```python
from build123d import *

# Parameters (mm, degrees)
SKETCH_W        = 12
SKETCH_H        = 77
PAD_DEPTH       = 5
PAD001_DEPTH    = 5.1
PAD002_DEPTH    = 3
SKETCH003_W     = 4
SKETCH003_H     = 105
SKETCH003_W_2   = 10
SKETCH003_H_2   = 5
PAD003_DEPTH    = 12
SKETCH004_W     = 6
SKETCH004_H     = 10
POCKET_DEPTH    = 3
POCKET001_DEPTH = 12.001
FILLET_R        = 2
PAD004_DEPTH    = 12
FILLET001_R     = 2
CHAMFER_SIZE    = 1


with BuildPart() as part:
    # Sketch → Pad (new body)
    with BuildSketch(Plane.XZ):
        with Locations((0, 38.5)):
            Rectangle(SKETCH_W, SKETCH_H)
    extrude(amount=PAD_DEPTH)

    # Sketch001 (on Face6 of Pad) → Pad001 (join)
    with BuildSketch(Plane.XZ.offset(5)):
        with BuildLine():
            Line((-2.2, 25.05), (-2.2, 22.45))
            ThreePointArc((-2.2, 22.45), (0, 20.25), (2.2, 22.45))
            Line((2.2, 25.05), (2.2, 22.45))
            ThreePointArc((2.2, 25.05), (0, 27.25), (-2.2, 25.05))
        make_face()
        with BuildLine():
            Line((-2.2, 65.05), (-2.2, 62.45))
            ThreePointArc((-2.2, 62.45), (0, 60.25), (2.2, 62.45))
            Line((2.2, 65.05), (2.2, 62.45))
            ThreePointArc((2.2, 65.05), (0, 67.25), (-2.2, 65.05))
        make_face()
    extrude(amount=PAD001_DEPTH)

    # Sketch002 (on Face16 of Pad001) → Pad002 (join)
    with BuildSketch(Plane.XZ.offset(10.1)):
        with BuildLine():
            Line((-2.2, 25.05), (-2.2, 16.45))
            ThreePointArc((-2.2, 16.45), (0, 14.25), (2.2, 16.45))
            Line((2.2, 25.05), (2.2, 16.45))
            ThreePointArc((2.2, 25.05), (0, 27.25), (-2.2, 25.05))
        make_face()
        with BuildLine():
            Line((-2.2, 65.05), (-2.2, 56.45))
            ThreePointArc((-2.2, 56.45), (0, 54.25), (2.2, 56.45))
            Line((2.2, 65.05), (2.2, 56.45))
            ThreePointArc((2.2, 65.05), (0, 67.25), (-2.2, 65.05))
        make_face()
    extrude(amount=PAD002_DEPTH)

    # Sketch003 (on Face6 of Pad002) → Pad003 (join)
    with BuildSketch(Plane(origin=(6, 0, 0), x_dir=(0, 0, 1), z_dir=(1, 0, 0))):
        with Locations((2, -52.5)):
            Rectangle(SKETCH003_W, SKETCH003_H)
        with Locations((9, -12.5)):
            Rectangle(SKETCH003_W_2, SKETCH003_H_2)
        with Locations((9, -27.5)):
            Rectangle(SKETCH003_W_2, SKETCH003_H_2)
        with Locations((9, -42.5)):
            Rectangle(SKETCH003_W_2, SKETCH003_H_2)
        with Locations((9, -57.5)):
            Rectangle(SKETCH003_W_2, SKETCH003_H_2)
        with Locations((9, -72.5)):
            Rectangle(SKETCH003_W_2, SKETCH003_H_2)
        with Locations((9, -87.5)):
            Rectangle(SKETCH003_W_2, SKETCH003_H_2)
        with Locations((9, -102.5)):
            Rectangle(SKETCH003_W_2, SKETCH003_H_2)
    extrude(amount=-PAD003_DEPTH)

    # Sketch004 (on Face30 of Pad003) → Pocket (cut)
    with BuildSketch(Plane(origin=(0, 0, 4), x_dir=(-1, 0, 0), z_dir=(0, 0, 1))):
        with Locations((0, -5)):
            Rectangle(SKETCH004_W, SKETCH004_H)
        with Locations((0, -20)):
            Rectangle(SKETCH004_W, SKETCH004_H)
        with Locations((0, -35)):
            Rectangle(SKETCH004_W, SKETCH004_H)
        with Locations((0, -50)):
            Rectangle(SKETCH004_W, SKETCH004_H)
        with Locations((0, -65)):
            Rectangle(SKETCH004_W, SKETCH004_H)
        with Locations((0, -80)):
            Rectangle(SKETCH004_W, SKETCH004_H)
        with Locations((0, -95)):
            Rectangle(SKETCH004_W, SKETCH004_H)
    extrude(amount=-POCKET_DEPTH, mode=Mode.SUBTRACT)

    # Sketch005 (on Face5 of Pocket) → Pocket001 (cut, through all)
    with BuildSketch(Plane(origin=(6, 0, 0), x_dir=(0, 0, 1), z_dir=(1, 0, 0))):
        with BuildLine():
            ThreePointArc((74.499999, 0), (77, 2.5), (74.5, 5))
            Line((74.5, 5), (77.1, 5))
            Line((77.1, 5), (77.099999, 0))
            Line((74.499999, 0), (77.099999, 0))
        make_face()
    extrude(amount=-POCKET001_DEPTH, mode=Mode.SUBTRACT)

    # Fillet
    fillet_edges = [part.edges().sort_by_distance(p)[0] for p in [
        (0, 105, 14),
        (0, 100, 14),
        (0, 90, 14),
        (0, 85, 14),
        (0, 75, 14),
        (0, 70, 14),
        (0, 60, 14),
        (0, 55, 14),
        (0, 45, 14),
        (0, 40, 14),
        (0, 30, 14),
        (0, 25, 14),
        (0, 15, 14),
        (0, 10, 14),
    ]]
    fillet(fillet_edges, radius=FILLET_R)

    # Sketch006 (on Face5 of Fillet) → Pad004 (join)
    with BuildSketch(Plane(origin=(6, 0, 0), x_dir=(0, 0, 1), z_dir=(1, 0, 0))):
        Polygon((-12, 5), (0, 5), (0, -105), align=None)
    extrude(amount=-PAD004_DEPTH)

    # Fillet001
    fillet001_edges = [part.edges().sort_by_distance(p)[0] for p in [
        (0, 105, 0),
        (0, -5, -12),
    ]]
    fillet(fillet001_edges, radius=FILLET001_R)

    # Chamfer
    chamfer_edges = [part.edges().sort_by_distance(p)[0] for p in [
        (6, -5, 32.365024),
        (6, -4.33533, -11.258877),
        (6, -4.267767, 76.267767),
        (6, 50.216895, -5.976339),
        (6, -0.732233, 76.267767),
        (6, 104.488924, 0.458354),
        (6, 0, 39.25),
        (6, 105, 6.896842),
        (6, 5, 4),
        (6, 104.414214, 13.414214),
        (6, 10, 8),
        (6, 102.5, 14),
        (6, 10.585786, 13.414214),
        (6, 100.585786, 13.414214),
        (6, 12.5, 14),
        (6, 100, 8),
        (6, 14.414214, 13.414214),
        (6, 95, 4),
        (6, 15, 8),
        (6, 90, 8),
        (6, 20, 4),
        (6, 89.414214, 13.414214),
        (6, 25, 8),
        (6, 87.5, 14),
        (6, 25.585786, 13.414214),
        (6, 85.585786, 13.414214),
        (6, 27.5, 14),
        (6, 85, 8),
        (6, 29.414214, 13.414214),
        (6, 80, 4),
        (6, 30, 8),
        (6, 75, 8),
        (6, 35, 4),
        (6, 74.414214, 13.414214),
        (6, 40, 8),
        (6, 72.5, 14),
        (6, 40.585786, 13.414214),
        (6, 70.585786, 13.414214),
        (6, 42.5, 14),
        (6, 70, 8),
        (6, 44.414214, 13.414214),
        (6, 65, 4),
        (6, 45, 8),
        (6, 60, 8),
        (6, 50, 4),
        (6, 59.414214, 13.414214),
        (6, 55, 8),
        (6, 57.5, 14),
        (6, 55.585786, 13.414214),
        (-6, 105, 6.896842),
        (-6, 104.488924, 0.458354),
        (-6, 104.414214, 13.414214),
        (-6, 50.216895, -5.976339),
        (-6, 102.5, 14),
        (-6, -4.33533, -11.258877),
        (-6, 100.585786, 13.414214),
        (-6, -5, 32.365024),
        (-6, 100, 8),
        (-6, -4.267767, 76.267767),
        (-6, 95, 4),
        (-6, -0.732233, 76.267767),
        (-6, 90, 8),
        (-6, 0, 39.25),
        (-6, 89.414214, 13.414214),
        (-6, 5, 4),
        (-6, 87.5, 14),
        (-6, 10, 8),
        (-6, 85.585786, 13.414214),
        (-6, 10.585786, 13.414214),
        (-6, 85, 8),
        (-6, 12.5, 14),
        (-6, 80, 4),
        (-6, 14.414214, 13.414214),
        (-6, 75, 8),
        (-6, 15, 8),
        (-6, 74.414214, 13.414214),
        (-6, 20, 4),
        (-6, 72.5, 14),
        (-6, 25, 8),
        (-6, 70.585786, 13.414214),
        (-6, 25.585786, 13.414214),
        (-6, 70, 8),
        (-6, 27.5, 14),
        (-6, 65, 4),
        (-6, 29.414214, 13.414214),
        (-6, 60, 8),
        (-6, 30, 8),
        (-6, 59.414214, 13.414214),
        (-6, 35, 4),
        (-6, 57.5, 14),
        (-6, 40, 8),
        (-6, 55.585786, 13.414214),
        (-6, 40.585786, 13.414214),
        (-6, 55, 8),
        (-6, 42.5, 14),
        (-6, 50, 4),
        (-6, 44.414214, 13.414214),
        (-6, 45, 8),
    ]]
    chamfer(chamfer_edges, length=CHAMFER_SIZE)


solid = part.part
```
Here's how the part is built. I have some questions about the finished solid (model axes, mm). A direction names the side the tool comes from. Give positions to 0.01 mm unless a question says otherwise; leave off trailing zeros. Loops run counter-clockwise (first coordinate to the right, second up) from the corner with the lowest first, then second, coordinate; pieces in that order, holes last. Notation, with made-up numbers: M 7.25,14 L 59.25,14 A21 ccw 59.25,45 Z; hole C 79.25,-9 d9. An arc over 180 degrees is marked long. Return JSON: item names as keys, results as strings.
Item 1: Please list where these lines run through material, in increasing order: line 1 (Y direction, x = 0, z = 20.5); line 2 (Y direction, x = 3.25, z = 36.5); line 3 (Z direction, x = -1.75, y = 92.5).
A:
{"line 1": "y = -13.1 to 0", "line 2": "y = -5 to 0", "line 3": "z = -1.36 to 1"}
Item 2: Imagine slicing it at A-A on z = 30. List the corners of the cut face in (x, y) for me, then the cut area to 3 significant figures.
A:
{"outline": "M -6,-4 L -5,-5 L 5,-5 L 6,-4 L 6,-1 L 5,0 L -5,0 L -6,-1 Z", "area": "58.0 mm^2"}
Item 3: Imagine slicing it at D-D on y = 6. List the corners of the cut face in (x, z) for me.
A:
{"outline": "M -6,-9.79 L -5,-10.8 L 5,-10.8 L 6,-9.79 L 6,3 L 5,4 L 3,4 L 3,1 L -3,1 L -3,4 L -5,4 L -6,3 Z"}
Item 4: Imagine slicing it at C-C on z = -4. List the corners of the cut face in (x, y) for me.
A:
{"outline": "M -6,-4 L -5,-5 L 5,-5 L 6,-4 L 6,59.11 L 5,68.33 L -5,68.33 L -6,59.11 Z"}
Item 5: I'm going to push flat-ended pins straight in: pin 1 Ø5 at (x, z) = (-4, 29.5) entering from -Y; pin 2 Ø1 at (x, y) = (3, -1) entering from -Z; pin 3 Ø1.5 at (x, y) = (3.5, 44) entering from -Z. Where does each tip first touch, or does it pass through?
A:
{"pin 1": "stops at y = -5", "pin 2": "stops at z = -11.62", "pin 3": "stops at z = -6.74"}
Item 6: On a 3-axis mill with a long thin cutter (end or side, diameter ignored), from which of +Z, -Z, +X, -X, +Y, -Y can I reach the whole of each face in a straight line? I mean faces 1 (the cylindrical face through (0.05, -8.99, 27.25)), 2 (the flat face through (-6, 30, 1)), 3 (the flat face through (-2.2, -11, 22)), 4 (the conical face through (-5.8, -2.5, 76.2)), 5 (the flat face through (0, 65, 1)). Say none if no direction works.
A:
{"face 1": "-Y", "face 2": "+Z, -Z, -X, +Y, -Y", "face 3": "+Z, -Z, -X, -Y", "face 4": "+Z, -X", "face 5": "+Z"}
Item 7: Thinking about a two-plate mould opening in Y: for faces 6 (the flat face through (0, 25, 8)), 7 (the cylindrical face through (-0.05, -11.58, 14.25)), 8 (the flat face through (0.07, 50.959, -5.895)), which applies, released by +Y, released by -Y, zero draft, split by the parting line, or undercut?
A:
{"face 6": "undercut", "face 7": "zero draft", "face 8": "released by +Y"}
Item 8: Imagine slicing it at B-B on y = 67. List the corners of the cut face in (x, z) for me, then the cut area to 3 significant figures.
A:
{"outline": "M -6,-3.14 L -5,-4.15 L 5,-4.15 L 6,-3.14 L 6,3 L 5,4 L 3,4 L 3,1 L -3,1 L -3,4 L -5,4 L -6,3 Z", "area": "77.7 mm^2"}
